Autodesk Inventor part; units mm, degrees
ref_plane "YZ Plane" through (0, 0, 0) normal (1, 0, 0) x (0, 1, 0)
ref_plane "XZ Plane" through (0, 0, 0) normal (0, 1, 0) x (-1, 0, 0)
ref_plane "XY Plane" through (0, 0, 0) normal (0, 0, 1) x (1, 0, 0)
sketch "Sketch1" plane through (0, 0, 0) normal (0, 0, 1) x (1, 0, 0)
  line L0 (0, 0) -> (12, 0)
  line L1 (12, 0) -> (12, 30)
  line L2 (12, 30) -> (0, 30)
  line L3 (0, 30) -> (0, 0)
  dimension "d0" = 12
  dimension "d1" = 30
extrude "Extrusion1" add sketch "Sketch1" along normal blind 13.0302
sketch "Sketch2" plane through (0, 0, 13.0302) normal (0, 0, 1) x (1, 0, 0)
  line L0 (12, 30) -> (0, 30)
  line L1 (0, 30) -> (0, 0)
  circle A0 centre (6, 21.11) radius 3.5052
  dimension "d4" = 6
  dimension "d5" = 8.89
  dimension "d8" = 7.0104
extrude "Extrusion2" add sketch "Sketch2" along normal blind 3.175
equation "\"d0\" = servoWidth"
equation "\"d1\" = servoLength"
equation "\"d2\" = servoHeight"
equation "\"d4\" = 0.5 * servoWidth"
equation "\"d5\" = hornOffset"
equation "\"d8\" = hornCenter"
equation "\"d6\" = thick"
equation "\"servoLength\" = 30"
equation "\"servoWidth\" = 12"
equation "\"hornCenter\" = 7.0104"
equation "\"hornDia\" = 13.1572"
equation "\"hornHole\" = 1.524"
equation "\"hornOffset\" = 8.89"
equation "\"servoHeight\" = 13.0302"
equation "\"thick\" = 3.175"
properties part number "Servo"
Source: CAD feature listing. Evaluate the final solid. Frame: model axes, mm. A direction names the side the tool comes from. Coordinates: 2 decimals unless noted, no trailing zeros. Loops run counter-clockwise (first coordinate to the right, second up) from the corner with the lowest first, then second, coordinate; pieces in that order, holes last. Notation, with made-up numbers: (45.25, 86.5) -> (60.25, 86.5) arc R28 ccw to (60.25, 124.5) -> close; hole circle Ø7 at (0, -10). An arc over 180 degrees is marked (long way). Answer in a Markdown table with one row per item. Add a question column.
Q1. Ray query, line 1 along Z through (x, y) = (4.75, 4.75); line 2 along Y through (x, z) = (7.5, 13.5). Return the intervals inside material, ascending.
Q2. Contact query for flat-ended pins moving along their axis: pin 1 Ø1 at (x, y) = (1.5, 10.5) entering from +Z; pin 2 Ø4 at (x, z) = (8.5, 13.5) entering from -Y. Output: stop coordinate, or through.
Q3. Section A-A on x = 6. Return the cut outline in (y, z).
Q4. Reachability of faces 1 (the face through (12, 15, 6)), 2 (the face through (5.24, 24.53, 14.6)) from +Z, -Z, +X, -X, +Y, -Y: full face, straight path, thin tool, end or side. Return the list, or none.
Q5. Section C-C on z = 13.5. Return the cut outline in (x, y).
Q6. Section D-D on x = 10.75. Return the cut outline in (y, z).
Q7. Section B-B on y = 21.11. Return the cut outline in (x, z).
Computed values:
| question | item | result |
|---|---|---|
| 1 | line 1 | z = 0 to 13.03 |
| 1 | line 2 | y = 17.94 to 24.28 |
| 2 | pin 1 | stops at z = 13.03 |
| 2 | pin 2 | stops at y = 0 |
| 3 | outline | (0, 0) -> (30, 0) -> (30, 13.03) -> (24.62, 13.03) -> (24.62, 16.21) -> (17.6, 16.21) -> (17.6, 13.03) -> (0, 13.03) -> close |
| 4 | face 1 | +Z, -Z, +X, +Y, -Y |
| 4 | face 2 | +Z |
| 5 | outline | circle Ø7.01 at (6, 21.11) |
| 6 | outline | (0, 0) -> (30, 0) -> (30, 13.03) -> (0, 13.03) -> close |
| 7 | outline | (0, 0) -> (12, 0) -> (12, 13.03) -> (9.51, 13.03) -> (9.51, 16.21) -> (2.49, 16.21) -> (2.49, 13.03) -> (0, 13.03) -> close |
